Check sheet for the modelled part. Datum: model origin and axes. Units: mm. Coordinates: 2 decimals unless noted, no trailing zeros. Loops run counter-clockwise (first coordinate to the right, second up) from the corner with the lowest first, then second, coordinate; pieces in that order, holes last. Notation, with made-up numbers: (66, 83.5) -> (78, 83.5) arc R17 ccw to (78, 87.5) -> close; hole circle Ø7 at (4, 6). An arc over 180 degrees is marked (long way). Use CSV: the item, a comma, the result in double quotes. Start each with the question number.
1. Release check for a two-part mould opening along Y. For faces 1 (the face through (-12.756, 21, -58)), 2 (the face through (-27.9, 1, -58)), 3 (the face through (15.016, 15.458, -57.703)), 4 (the face through (-7.33, 21.05, -57.66)) record: pulls with the +Y half, pulls with the -Y half, needs draft (parallel to the pull), parting line crosses it, or undercut.
2. Gauge pin test, flat ends, axial feed: pin 1 (1.5 mm diameter, centred on x = -11, z = -58, fed in from -Y); pin 2 (2.5 mm diameter, centred on x = -5.9, y = 20.6, fed in from +Z); pin 3 (0.8 mm diameter, centred on y = 20.5, z = -57.5, fed in from +X); pin 4 (0.8 mm diameter, centred on y = 20.5, z = -58, fed in from -X). Record the tip position at first contact, or that the pin passes through.
3. Sectioned sample at A-A, the plane x = -0.5. Record the cut outline in (y, z).
4. Sectioned sample at C-C, the plane z = -56.9. Count the separate pieces of the cut face and the enclosed holes in it, and give its area (3 significant figures).
5. Sectioned sample at B-B, the plane y = 4.5. Record the cut outline in (x, z), and give its area (3 significant figures).
6. Thickness scan on L1, parallel to Y at x = -5.9, z = -58.3; L2, parallel to X at y = 10, z = -58.8; L3, parallel to Y at x = 9.5, z = -57.55. Record the ranges inside material, lowest first.
```python
from build123d import *

# Parameters (mm, degrees)
SKETCH_R                 = 1.5
SKETCH_W                 = 2.700009
SKETCH_H                 = 2.699989
PAD_DEPTH                = 3
FILLET_R                 = 3.8
FILLET001_R              = 11.8
CLONE003_PLACEMENT_ANGLE = 180


with BuildPart() as part:
    # Sketch (on Face9 of Binder004) → Pad (new body)
    with BuildSketch(Plane(origin=(0, 1.8e-05, 2.818036), x_dir=(1, 0, 0), z_dir=(0, -6e-06, -1))):
        Polygon((-30, 24.600493), (-30, -15.399507), (-22, -15.399507), (-22, 16.600493), (22, 16.600493), (22, -15.399507), (30, -15.399507), (30, 24.600493), align=None)
        with Locations((0, 20.600493)):
            Circle(SKETCH_R, mode=Mode.SUBTRACT)
        with Locations((-5.49402, 20.600472)):
            Rectangle(SKETCH_W, SKETCH_H, mode=Mode.SUBTRACT)
        with Locations((5.50598, 20.600513)):
            Rectangle(SKETCH_W, SKETCH_H, mode=Mode.SUBTRACT)
    extrude(amount=PAD_DEPTH)

    # Fillet
    fillet_edges = [part.edges().sort_by_distance(p)[0] for p in [
        (-30, 15.399516, 1.317937),
        (-22, 15.399516, 1.317937),
        (22, 15.399516, 1.317937),
        (30, 15.399516, 1.317937),
        (-22, -16.600484, 1.318144),
        (22, -16.600484, 1.318144),
    ]]
    fillet(fillet_edges, radius=FILLET_R)

    # Fillet001
    fillet001_edges = [part.edges().sort_by_distance(p)[0] for p in [
        (30, -24.600484, 1.318195),
        (-30, -24.600484, 1.318195),
    ]]
    fillet(fillet001_edges, radius=FILLET001_R)


with BuildPart() as part_1:
    # Body placement: moved
    add(part.part.moved(Location((12.1, 0, -69.4))))


with BuildPart() as part_2:
    # Clone003 placement: moved
    add(part_1.part.moved(Location((6.2, 0, 10.4))).rotate(Axis((6.2, 0, 10.4), (0, 0, 1)), CLONE003_PLACEMENT_ANGLE))


solid = part_2.part
```
Completed:
1,face 1,"undercut"
1,face 2,"needs draft"
1,face 3,"pulls with the -Y half"
1,face 4,"undercut"
2,pin 1,"y = 16.6"
2,pin 2,"through"
2,pin 3,"x = 21.57"
2,pin 4,"x = -33.37"
3,outline,"(16.6, -59.18) -> (19.25, -59.18) -> (19.25, -56.18) -> (16.6, -56.18) -> close; (21.95, -59.18) -> (24.6, -59.18) -> (24.6, -56.18) -> (21.95, -56.18) -> close"
4,separate pieces,"1"
4,enclosed holes,"3"
4,area,"904 mm²"
5,outline,"(-35.9, -59.18) -> (-27.9, -59.18) -> (-27.9, -56.18) -> (-35.9, -56.18) -> close; (16.1, -59.18) -> (24.1, -59.18) -> (24.1, -56.18) -> (16.1, -56.18) -> close"
5,area,"48.0 mm²"
6,L1,"16.6 to 19.1, 22.1 to 24.6"
6,L2,"-35.9 to -27.9, 16.1 to 24.1"
6,L3,"16.6 to 24.6"
